Here's how the part is built. I have some questions about the finished solid (model axes, mm). A direction names the side the tool comes from. Round coordinates to 2 decimals unless told otherwise and drop trailing zeros. Order: outer loops, then holes, each group sorted by start corner. A loop starts at its lowest first (then second) coordinate and runs counter-clockwise, first axis right, second up. Notation, with made-up numbers: (62.5, 43.5) -> (75.5, 43.5) arc R20 ccw to (75.5, 77.5) -> close; hole circle Ø11 at (37.25, 85.25). An arc over 180 degrees is marked (long way). Answer in a Markdown table with one row per item.
```python
from build123d import *

# Parameters (mm, degrees)
F1_R      = 6.35
F2_DEPTH  = 12.7
F4_DEPTH  = 12.701
F8_R      = 2.54
F10_DEPTH = 6.35
F9_R      = 6.35
F11_DEPTH = 89.8035612107


with BuildPart() as f2:
    # F1 (on Top) → F2 (new body)
    with BuildSketch(Plane.XY):
        with BuildLine():
            ThreePointArc((-31.75, 31.75), (-44.45, 44.45), (-57.15, 31.75))
            Line((-57.15, 31.75), (-57.15, 6.35))
            Line((-57.15, 6.35), (-44.45, 6.35))
            ThreePointArc((-44.45, 6.35), (-38.1, 0), (-44.45, -6.35))
            Line((-44.45, -6.35), (-57.15, -6.35))
            Line((-57.15, -6.35), (-57.15, -31.75))
            ThreePointArc((-57.15, -31.75), (-44.45, -44.45), (-31.75, -31.75))
            Line((-31.75, -31.75), (-31.75, -25.4))
            Line((-31.75, -25.4), (31.75, -25.4))
            Line((31.75, -25.4), (31.75, -31.75))
            ThreePointArc((31.75, -31.75), (44.45, -44.45), (57.15, -31.75))
            Line((57.15, -31.75), (57.15, 31.75))
            ThreePointArc((57.15, 31.75), (44.45, 44.45), (31.75, 31.75))
            Line((31.75, 31.75), (31.75, 25.4))
            Line((31.75, 25.4), (-31.75, 25.4))
            Line((-31.75, 25.4), (-31.75, 31.75))
        make_face()
        with Locations((-44.45, -31.75)):
            Circle(F1_R, mode=Mode.SUBTRACT)
        with Locations((44.45, -31.75)):
            Circle(F1_R, mode=Mode.SUBTRACT)
        with Locations((-44.45, 31.75)):
            Circle(F1_R, mode=Mode.SUBTRACT)
        with Locations((44.45, 31.75)):
            Circle(F1_R, mode=Mode.SUBTRACT)
        with Locations((-44.45, -31.75)):
            Circle(F1_R)
        with Locations((-44.45, 31.75)):
            Circle(F1_R)
        with Locations((44.45, 31.75)):
            Circle(F1_R)
        with Locations((44.45, -31.75)):
            Circle(F1_R)
    extrude(amount=-F2_DEPTH)

    # F1 (on Top) → F4 (cut, through all)
    with BuildSketch(Plane.XY):
        with Locations((-44.45, -31.75)):
            Circle(F1_R)
        with Locations((-44.45, 31.75)):
            Circle(F1_R)
        with Locations((44.45, 31.75)):
            Circle(F1_R)
        with Locations((44.45, -31.75)):
            Circle(F1_R)
    extrude(amount=-F4_DEPTH, mode=Mode.SUBTRACT)

    # F6 (on face) → F7 (join, up to the next surface of F2)
    with BuildSketch(Plane(origin=(28.575, 0, 28.575), x_dir=(0.7071067812, 0, -0.7071067812), z_dir=(-0.7071067812, 0, -0.7071067812))):
        with BuildLine():
            Line((40.4111525448, -25.4), (40.4111525448, 25.4))
            Line((40.4111525448, 25.4), (8.6611525448, 25.4))
            ThreePointArc((8.6611525448, 25.4), (-16.7388474552, 0), (8.6611525448, -25.4))
            Line((8.6611525448, -25.4), (40.4111525448, -25.4))
        make_face()
    extrude(until=Until.NEXT)

    # F8 (on face) → F10 (cut)
    with BuildSketch(Plane(origin=(28.575, 0, 28.575), x_dir=(0.7071067812, 0, -0.7071067812), z_dir=(-0.7071067812, 0, -0.7071067812))):
        with Locations((-10.3888474552, 0)):
            Circle(F8_R)
        with Locations((-1.6133632838, -12.0784177569)):
            Circle(F8_R)
        with Locations((12.5856683734, -7.4648727041)):
            Circle(F8_R)
        with Locations((12.5856683734, 7.4648727041)):
            Circle(F8_R)
        with Locations((-1.6133632838, 12.0784177569)):
            Circle(F8_R)
    extrude(amount=F10_DEPTH, mode=Mode.SUBTRACT)

    # F9 (on face) → F11 (cut, through all)
    with BuildSketch(Plane(origin=(28.575, 0, 28.575), x_dir=(0.7071067812, 0, -0.7071067812), z_dir=(-0.7071067812, 0, -0.7071067812))):
        with Locations((2.3111525448, 0)):
            Circle(F9_R)
    extrude(amount=F11_DEPTH, mode=Mode.SUBTRACT)


solid = f2.part
```
1. Suppose I cut it at D-D on x = -28.5. Write out the boundary of the cut face in (y, z).
Numbers:
| item | result |
|---|---|
| outline | (-25.4, -12.7) -> (25.4, -12.7) -> (25.4, 0) -> (-25.4, 0) -> close |
2. Suppose I cut it at C-C on x = 49. Write out the boundary of the cut face in (y, z).
Numbers:
| item | result |
|---|---|
| outline | (-43.61, -12.7) -> (-36.18, -12.7) -> (-36.18, 0) -> (-43.61, 0) -> close; (-27.32, -12.7) -> (27.32, -12.7) -> (27.32, 0) -> (25.4, 0) -> (25.4, 8.15) -> (-25.4, 8.15) -> (-25.4, 0) -> (-27.32, 0) -> close; (36.18, -12.7) -> (43.61, -12.7) -> (43.61, 0) -> (36.18, 0) -> close |
3. Suppose I cut it at A-A on x = -42.5. Write out the boundary of the cut face in (y, z).
Numbers:
| item | result |
|---|---|
| outline | (-44.3, -12.7) -> (-37.79, -12.7) -> (-37.79, 0) -> (-44.3, 0) -> close; (-25.71, -12.7) -> (-6.04, -12.7) -> (-6.04, 0) -> (-25.71, 0) -> close; (6.04, -12.7) -> (25.71, -12.7) -> (25.71, 0) -> (6.04, 0) -> close; (37.79, -12.7) -> (44.3, -12.7) -> (44.3, 0) -> (37.79, 0) -> close |
4. For pin 1 Ø4 at (x, z) = (-47.5, -9) entering from -Y; pin 2 Ø5 at (x, y) = (-34.5, 34.5) entering from +Z; pin 3 Ø2 at (x, z) = (0, 1.5) entering from -Y, each with a flat end and sliding along its axis, tell me the tip position at first contact or that it passes through.
Numbers:
| item | result |
|---|---|
| pin 1 | stops at y = -44.41 |
| pin 2 | stops at z = 0 |
| pin 3 | stops at y = -23.86 |
5. Please list where these lines run through material, in increasing order: line 1 along Y through (x, z) = (44, -3); line 2 along Y through (x, z) = (-44, -8); line 3 along X through (y, z) = (33.5, -8.5).
Numbers:
| item | result |
|---|---|
| line 1 | y = -44.44 to -38.08, -25.42 to 25.42, 38.08 to 44.44 |
| line 2 | y = -44.44 to -38.08, -25.42 to -6.33, 6.33 to 25.42, 38.08 to 44.44 |
| line 3 | x = -57.03 to -50.55, -38.35 to -31.87, 31.87 to 38.35, 50.55 to 57.03 |
6. Suppose I cut it at B-B on y = -30. Write out the boundary of the cut face in (x, z), then the cut area to 3 significant figures.
Numbers:
| item | result |
|---|---|
| outline | (-57.15, -12.7) -> (-50.55, -12.7) -> (-50.55, 0) -> (-57.15, 0) -> close; (-38.35, -12.7) -> (-31.75, -12.7) -> (-31.75, 0) -> (-38.35, 0) -> close; (31.75, -12.7) -> (38.35, -12.7) -> (38.35, 0) -> (31.75, 0) -> close; (50.55, -12.7) -> (57.15, -12.7) -> (57.15, 0) -> (50.55, 0) -> close |
| area | 335 mm2 |
7. For faces 4 (the face through (44, -39, 0)), 5 (the face through (-51, -6.35, -6)), 6 (the face through (50.507, 33.657, -6.261)), 7 (the face through (15, -25.4, 2)), 8 (the face through (22.92, 12.04, 25.25)), which set-ups out of +Z, -Z, +X, -X, +Y, -Y let a thin tool reach every point of the face, with its end or its side?
Numbers:
| item | result |
|---|---|
| face 4 | +Z, +X, -X, -Y |
| face 5 | +Z, -Z, -X |
| face 6 | +Z, -Z |
| face 7 | +Z, -Y |
| face 8 | none |
8. We'd pull the mould along Z, two halves only. Please class faces 1 (the face through (-31.75, -29, -6)), 2 (the face through (23.897, -13.795, 28.826)), 3 (the face through (44, 39, 0)): released by +Z, released by -Z, zero draft, split by the parting line, or undercut.
Numbers:
| item | result |
|---|---|
| face 1 | zero draft |
| face 2 | undercut |
| face 3 | released by +Z |
